Part model, mm, in its own coordinate system. A direction names the side the tool comes from. Give positions to 0.01 mm unless a question says otherwise; leave off trailing zeros. Write each loop counter-clockwise with the first axis right and the second up, starting at its lowest first coordinate (ties: lowest second). Pieces come first, ordered by that corner, then holes. Notation, with made-up numbers: (73, 6) - (95, 6) arc R11 ccw to (95, 14) - close; hole circle Ø9 at (66.5, 28). An arc over 180 degrees is marked (long way). Answer in a Markdown table with one row per item. Add a question column.
1. Band-saw the part on B-B on y = -65.75. State how many separate pieces and enclosed holes the cut face has, plus the area to 3 significant figures.
2. Band-saw the part on A-A on x = 37.2. Write the cut outline in (y, z).
3. Band-saw the part on C-C on x = 16.5. Write the cut outline in (y, z), plus the area to 3 significant figures.
4. Pull direction X, two halves, no side cores. Call faces 1 (the cylindrical face through (-12.5, -64.98, 39.15)), 2 (the cylindrical face through (58.62, -62.18, 15.71)), 3 (the flat face through (55.576, -62.995, 50.274)): released by +X, released by -X, zero draft, split by the parting line, or undercut.
5. Band-saw the part on D-D on x = -35. Write the cut outline in (y, z) (3 decimals).
6. Which spindle directions (+Z, -Z, +X, -X, +Y, -Y) get a long thin tool onto all of the face, cutting with end or side? Do faces 4 (the flat face through (-55.58, -62.97, 17.77)), 5 (the flat face through (59.85, -60, 19)), 6 (the flat face through (-1, -65, 56.5)). Say none if no direction does.
7. Probe line 1 along Z through (x, y) = (59.15, -59.95); line 2 along Z through (x, y) = (37.2, -68.6); line 3 along Z through (x, y) = (38.5, -63.5). List the from-to ranges inside material, lowest first.
8. Drop flat-ended pins along their axis: pin 1 Ø5 at (x, y) = (57, -57) entering from -Z; pin 2 Ø3 at (x, y) = (-8, -64) entering from +Z; pin 3 Ø6 at (x, z) = (-10.5, 19) entering from +Y; pin 4 Ø15 at (x, z) = (-12.4, 34) entering from -Y. Give the stop position or say it passes through.
```python
from build123d import *

# Parameters (mm, degrees)
SKETCH010_W     = 126
SKETCH010_H     = 68
PAD006_DEPTH    = 3
SKETCH011_W     = 6
SKETCH011_H     = 12
PAD007_DEPTH    = 13.5
SKETCH012_R     = 2.25
POCKET004_DEPTH = 122.851
POCKET005_DEPTH = 3.5
CHAMFER003_SIZE = 1
CHAMFER004_SIZE = 1
CHAMFER007_SIZE = 1
SKETCH024_R     = 2.65
SKETCH024_R_2   = 8.15
SKETCH024_W     = 7.05
SKETCH024_H     = 19.25
POCKET012_DEPTH = 16.501
POCKET013_DEPTH = 1
CHAMFER010_SIZE = 2
SKETCH026_R     = 8.4
SKETCH026_R_2   = 6.65
POCKET014_DEPTH = 1.5
CHAMFER011_SIZE = 0.35
CHAMFER012_SIZE = 0.3
SKETCH030_R     = 5.15
SKETCH030_R_2   = 2.65
PAD012_DEPTH    = 4
SKETCH031_W     = 10.3
SKETCH031_H     = 2
POCKET016_DEPTH = 4
PAD016_DEPTH    = 4
FILLET003_R     = 0.1


with BuildPart() as part:
    # Sketch010 → Pad006 (new body)
    with BuildSketch(Plane.XZ):
        with Locations((0, 34)):
            Rectangle(SKETCH010_W, SKETCH010_H)
    extrude(amount=PAD006_DEPTH)

    # Sketch011 (on Face5 of Pad006) → Pad007 (join)
    with BuildSketch(Plane(origin=(0, 0, 0), x_dir=(1, 0, 0), z_dir=(0, 1, 0))):
        with Locations((-56.85, -16)):
            Rectangle(SKETCH011_W, SKETCH011_H)
        with Locations((-56.85, -52)):
            Rectangle(SKETCH011_W, SKETCH011_H)
    pad007 = extrude(amount=PAD007_DEPTH)

    # Mirrored002: Pad007 across YZ
    add(pad007.mirror(Plane.YZ))

    # Sketch012 (on Face22 of Mirrored002) → Pocket004 (cut, through all)
    with BuildSketch(Plane(origin=(59.85, 0, 0), x_dir=(0, 0, 1), z_dir=(1, 0, 0))):
        with Locations((16, -7)):
            Circle(SKETCH012_R)
        with Locations((52, -7)):
            Circle(SKETCH012_R)
    extrude(amount=-POCKET004_DEPTH, mode=Mode.SUBTRACT)

    # Sketch013 (on Face10 of Pocket004) → Pocket005 (cut)
    with BuildSketch(Plane(origin=(-53.85, 0, 0), x_dir=(0, 0, 1), z_dir=(1, 0, 0))):
        Polygon((19.5, -9.020726), (19.5, -4.979274), (16, -2.958548), (12.5, -4.979274), (12.5, -9.020726), (16, -11.041452), align=None)
        Polygon((55.5, -9.020726), (55.5, -4.979274), (52, -2.958548), (48.5, -4.979274), (48.5, -9.020726), (52, -11.041452), align=None)
    pocket005 = extrude(amount=-POCKET005_DEPTH, mode=Mode.SUBTRACT)

    # Chamfer003
    chamfer003_edges = [part.edges().sort_by_distance(p)[0] for p in [
        (0, -3, 68),
        (63, -3, 34),
        (0, -3, 0),
        (-63, -3, 34),
    ]]
    chamfer(chamfer003_edges, length=CHAMFER003_SIZE)

    # Chamfer004
    chamfer004_edges = [part.edges().sort_by_distance(p)[0] for p in [
        (-63, -1, 68),
        (63, -1, 68),
    ]]
    chamfer(chamfer004_edges, length=CHAMFER004_SIZE)

    # Chamfer007
    chamfer007_edges = [part.edges().sort_by_distance(p)[0] for p in [
        (63, -1, 0),
        (-63, -1, 0),
    ]]
    chamfer(chamfer007_edges, length=CHAMFER007_SIZE)

    # Mirrored005: Pocket005 across YZ
    add(pocket005.mirror(Plane.YZ), mode=Mode.SUBTRACT)

    # Sketch024 (on Face62 of Mirrored005) → Pocket012 (cut, through all)
    with BuildSketch(Plane.XZ.offset(3)):
        with Locations((-12.4, 34)):
            Circle(SKETCH024_R)
        with Locations((37.2, 34)):
            Circle(SKETCH024_R_2)
        with Locations((-37.2, 34)):
            Rectangle(SKETCH024_W, SKETCH024_H)
    extrude(amount=-POCKET012_DEPTH, mode=Mode.SUBTRACT)

    # Sketch025 (on Face1 of Pocket012) → Pocket013 (cut)
    with BuildSketch(Plane(origin=(0, 0, 0), x_dir=(1, 0, 0), z_dir=(0, 1, 0))):
        Polygon((-40.725, -20.375), (-33.675, -20.375), (-33.675, -43.625), (-33.675, -47.625), (-40.725, -47.625), (-40.725, -24.375), align=None)
    extrude(amount=-POCKET013_DEPTH, mode=Mode.SUBTRACT)

    # Chamfer010
    chamfer010_edges = [part.edges().sort_by_distance(p)[0] for p in [
        (-15.05, -3, 34),
    ]]
    chamfer(chamfer010_edges, length=CHAMFER010_SIZE)

    # Sketch026 (on Face4 of Chamfer010) → Pocket014 (cut)
    with BuildSketch(Plane.XZ.offset(3)):
        with Locations((-12.4, 34)):
            Circle(SKETCH026_R)
        with Locations((-12.4, 34)):
            Circle(SKETCH026_R_2, mode=Mode.SUBTRACT)
    extrude(amount=-POCKET014_DEPTH, mode=Mode.SUBTRACT)

    # Chamfer011
    chamfer011_edges = [part.edges().sort_by_distance(p)[0] for p in [
        (-19.05, -3, 34),
        (-20.8, -3, 34),
    ]]
    chamfer(chamfer011_edges, length=CHAMFER011_SIZE)

    # Chamfer012
    chamfer012_edges = [part.edges().sort_by_distance(p)[0] for p in [
        (-37.2, -3, 24.375),
        (-40.725, -3, 34),
        (-33.675, -3, 34),
        (-37.2, -3, 43.625),
        (29.05, -3, 34),
    ]]
    chamfer(chamfer012_edges, length=CHAMFER012_SIZE)

    # Sketch030 (on Face3 of Chamfer012) → Pad012 (join)
    with BuildSketch(Plane(origin=(0, 0, 0), x_dir=(1, 0, 0), z_dir=(0, 1, 0))):
        with Locations((-12.4, -34)):
            Circle(SKETCH030_R)
        with Locations((-12.4, -34)):
            Circle(SKETCH030_R_2, mode=Mode.SUBTRACT)
    extrude(amount=PAD012_DEPTH)

    # Sketch031 (on Face83 of Pad012) → Pocket016 (cut)
    with BuildSketch(Plane(origin=(0, 4, 0), x_dir=(1, 0, 0), z_dir=(0, 1, 0))):
        with Locations((-12.4, -34)):
            Rectangle(SKETCH031_W, SKETCH031_H)
    extrude(amount=-POCKET016_DEPTH, mode=Mode.SUBTRACT)

    # Sketch035 (on Face3 of Pocket016) → Pad016 (join)
    with BuildSketch(Plane(origin=(0, 0, 0), x_dir=(1, 0, 0), z_dir=(0, 1, 0))):
        with BuildLine():
            ThreePointArc((-40, -53.5), (-41.5, -55), (-40, -56.5))
            Line((-40, -56.5), (40, -56.5))
            ThreePointArc((40, -56.5), (41.5, -55), (40, -53.5))
            Line((-40, -53.5), (40, -53.5))
        make_face()
        with BuildLine():
            ThreePointArc((-40, -10.5), (-41.5, -12), (-40, -13.5))
            Line((-40, -13.5), (40, -13.5))
            ThreePointArc((40, -13.5), (41.5, -12), (40, -10.5))
            Line((-40, -10.5), (40, -10.5))
        make_face()
    extrude(amount=PAD016_DEPTH)

    # Fillet003
    fillet003_edges = [part.edges().sort_by_distance(p)[0] for p in [
        (-18.7, -3, 34),
        (-17.05, -3, 34),
    ]]
    fillet(fillet003_edges, radius=FILLET003_R)


with BuildPart() as part_1:
    # Body003 placement: moved
    add(part.part.moved(Location((0, -66.95, 0))))


solid = part_1.part
```
Values:
| question | item | result |
|---|---|---|
| 1 | separate pieces | 8 |
| 1 | enclosed holes | 0 |
| 1 | area | 833 mm² |
| 2 | outline | (-69.95, 1) - (-68.95, 0) - (-66.95, 0) - (-66.95, 10.5) - (-62.95, 10.5) - (-62.95, 13.5) - (-66.95, 13.5) - (-66.95, 25.85) - (-69.65, 25.85) - (-69.95, 25.55) - close; (-69.95, 42.45) - (-69.65, 42.15) - (-66.95, 42.15) - (-66.95, 53.5) - (-62.95, 53.5) - (-62.95, 56.5) - (-66.95, 56.5) - (-66.95, 68) - (-68.95, 68) - (-69.95, 67) - close |
| 3 | outline | (-69.95, 1) - (-68.95, 0) - (-66.95, 0) - (-66.95, 10.5) - (-62.95, 10.5) - (-62.95, 13.5) - (-66.95, 13.5) - (-66.95, 53.5) - (-62.95, 53.5) - (-62.95, 56.5) - (-66.95, 56.5) - (-66.95, 68) - (-68.95, 68) - (-69.95, 67) - close |
| 3 | area | 227 mm² |
| 4 | face 1 | split by the parting line |
| 4 | face 2 | zero draft |
| 4 | face 3 | undercut |
| 5 | outline | (-69.95, 1) - (-68.95, 0) - (-66.95, 0) - (-66.95, 10.5) - (-62.95, 10.5) - (-62.95, 13.5) - (-66.95, 13.5) - (-66.95, 20.375) - (-67.95, 20.375) - (-67.95, 24.375) - (-69.65, 24.375) - (-69.95, 24.075) - close; (-69.95, 43.925) - (-69.65, 43.625) - (-67.95, 43.625) - (-67.95, 47.625) - (-66.95, 47.625) - (-66.95, 53.5) - (-62.95, 53.5) - (-62.95, 56.5) - (-66.95, 56.5) - (-66.95, 68) - (-68.95, 68) - (-69.95, 67) - close |
| 6 | face 4 | none |
| 6 | face 5 | +Z, -Z, +X, +Y |
| 6 | face 6 | +Z, +Y |
| 7 | line 1 | z = 10 to 13.75, 18.25 to 22, 46 to 49.75, 54.25 to 58 |
| 7 | line 2 | z = 0 to 25.85, 42.15 to 68 |
| 7 | line 3 | z = 10.5 to 13.5, 53.5 to 56.5 |
| 8 | pin 1 | stops at z = 10 |
| 8 | pin 2 | stops at z = 56.5 |
| 8 | pin 3 | stops at y = -66.95 |
| 8 | pin 4 | stops at y = -69.95 |
